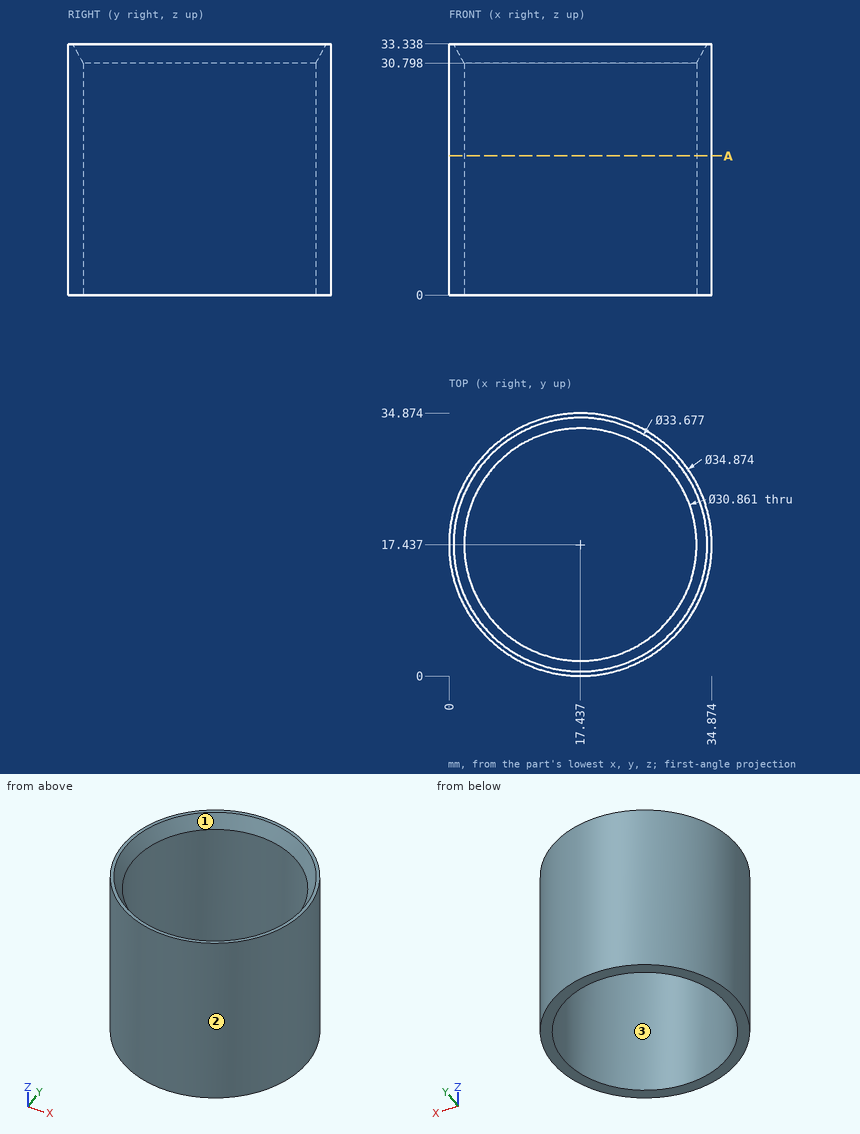
Input: dimensioned drawing with shaded views. Units: mm. Origin: part minimum x, y, z. Round coordinates to 2 decimals unless told otherwise and drop trailing zeros. Order: outer loops, then holes, each group sorted by start corner. A loop starts at its lowest first (then second) coordinate and runs counter-clockwise, first axis right, second up. Notation, with made-up numbers: (64.25, 26) - (100.25, 26) arc R29 cw to (100.25, 50) - close; hole circle Ø4 at (44.5, 58.5). An arc over 180 degrees is marked (long way). Write item = value, one per line. Start each with the question number.
Q1. Pull-direction query (Y, two-part tool) for the marked faces 1, 2 and 3; classes: +Y half, -Y half, draft (parallel to the pull), parting line (faces both ways), or undercut.
Q2. Cut plane A-A on z = 18.5. Return the cut outline in (x, y) (1 decimal), and give its area (3 significant figures).
Q3. Pin query (flat end, axial travel): pin 1 (1.5 mm diameter, centred on x = 26.5, z = 6, fed in from -Y); pin 2 (4 mm diameter, centred on y = 30.5, z = 15.5, fed in from -X); pin 3 (2 mm diameter, centred on y = 12.5, z = 10.5, fed in from +X); pin 4 (10 mm diameter, centred on x = 31, y = 18.5, fed in from -Z). Return the tip coordinate at first contact, or that it passes through.
Q4. Ray query, line 1 (Y direction, x = 18, z = 18.5) (1 decimal); line 2 (X direction, y = 10.5, z = 23) (1 decimal); line 3 (X direction, y = 15, z = 16) (1 decimal). Return the intervals inside material, ascending. Write a range as from..to.
Outcome:
q1.face_1 = undercut
q1.face_2 = parting line
q1.face_3 = undercut
q2.outline = circle Ø34.9 at (17.4, 17.4); hole circle Ø30.9 at (17.4, 17.4)
q2.area = 207 mm^2
q3.pin_1 = 2.11
q3.pin_2 = 3.96
q3.pin_3 = 34.42
q3.pin_4 = 0
q4.line_1 = 0..2, 32.9..34.9
q4.line_2 = 1.4..3.7, 31.2..33.4
q4.line_3 = 0.2..2.2, 32.7..34.7
